Part model, mm, in its own coordinate system. Round coordinates to 2 decimals unless told otherwise and drop trailing zeros. Order: outer loops, then holes, each group sorted by start corner. A loop starts at its lowest first (then second) coordinate and runs counter-clockwise, first axis right, second up. Notation, with made-up numbers: (-6.75, 0) - (42.25, 0) arc R11 cw to (42.25, 10) - close; hole circle Ø6 at (2, 62.5). An arc over 180 degrees is marked (long way). Return JSON: item names as keys, results as strings. Group by question number.
Item 1: Probe probe 1 along Y at (x, z) = (425.45, 0.5); probe 2 along Y at (x, z) = (361.95, 0.85); probe 3 along X at (y, z) = (-7, 1.15). List the from-to ranges inside material, lowest first.
Item 2: Saw through at D-D on x = 404. List the corners of the cut face in (y, z), and give its area (3 significant figures).
Item 3: Two-plate mould, pull along Y, no slides. Class faces 1 (the face through (364.155, -6.613, 0.783)), 2 (the face through (410, 13, 1.588)), 3 (the face through (450.57, -7.61, 0.78)): released by +Y, released by -Y, zero draft, split by the parting line, or undercut.
Item 4: Saw through at C-C on z = 1.2. List the corners of the cut face in (x, y), and give its area (3 significant figures).
Item 5: Saw through at B-B on y = 20.65. List the corners of the cut face in (x, z).
Item 6: Saw through at A-A on x = 425.45. List the corners of the cut face in (y, z), and give its area (3 significant figures).
Autodesk Inventor part; units mm, degrees
ref_plane "YZ Plane" through (0, 0, 0) normal (1, 0, 0) x (0, 1, 0)
ref_plane "XZ Plane" through (0, 0, 0) normal (0, 1, 0) x (-1, 0, 0)
ref_plane "XY Plane" through (0, 0, 0) normal (0, 0, 1) x (1, 0, 0)
sketch "Sketch1" plane through (0, 0, 0) normal (0, 0, 1) x (1, 0, 0)
  circle A0 centre (425.45, 20.65) radius 2.0828
  circle A1 centre (425.45, 20.65) radius 34.925 construction
  line L0 (425.45, 55.575) -> (298.45, 55.575) construction
  line L1 (323.85, 55.575) -> (323.85, 42.875) construction
  circle A2 centre (323.85, 12.649) radius 30.226 construction
  circle A3 centre (425.45, 20.65) radius 33.02 construction
  line L2 (406.9994, 48.5755) -> (348.6303, -5.5907)
  line L3 (420.1242, 27) -> (481.5758, 27)
  line L4 (442.214, -11.1) -> (383.027, -11.1)
  line L5 (450.1296, -1.1362) -> (416.5451, 47.5277)
  circle A4 centre (425.45, 20.65) radius 7.9375 construction
  arc A5 (416.5451, 47.5277) -> (406.9994, 48.5755) centre (411.3189, 43.9209) ccw
  line L6 (444.9034, -11.093) -> (350.7901, -11.093)
  line L7 (457.0011, -11.093) -> (551.1145, -11.093) construction
  arc A6 (444.9034, -11.093) -> (450.1296, -1.1362) centre (444.9034, -4.743) ccw
  arc A7 (348.6303, -5.5907) -> (350.7901, -11.093) centre (350.7901, -7.918) ccw
  circle A8 centre (387.35, -5.9184) radius 2.3114
  circle A9 centre (361.95, -5.9184) radius 2.3114
  circle A10 centre (438.15, -5.9184) radius 2.3114
  circle A11 centre (425.45, -5.9184) radius 2.3368
  point P0 (0, 0)
  point P1 (342.7011, -11.093)
  dimension "d0" = 69.85
  dimension "d1" = 127
  dimension "d2" = 12.7
  dimension "d3" = 60.452
  dimension "d4" = 30.226
  dimension "d5" = 101.6
  dimension "d6" = 66.04
  dimension "d9" = 15.875
  dimension "d10" = 6.35
  dimension "d11" = 180
  dimension "d12" = 114.3
  dimension "d13" = 6.35
  dimension "d14" = 3.175
  dimension "d15" = 5.1746
  dimension "d16" = 101.6
  dimension "d19" = 4.6736
  dimension "d20" = 12.7
extrude "Extrusion1" add sketch "Sketch1" along normal blind 1.5875 contours A5 L5 A6 L6 A7 L2 | A8 | A10 | A11
extrude "Extrusion2" cut sketch "Sketch1" along normal blind 1.5875 contours A11
properties part number "tangentsled"
Filled in:
{
 "1": {"probe 1": "y = -11.09 to -8.26, -3.58 to 18.57, 22.73 to 34.62", "probe 2": "y = -11.09 to -8.23, -3.61 to 6.77", "probe 3": "x = 347.75 to 359.91, 363.99 to 423.38, 427.52 to 450.84"},
 "2": {"outline": "(-11.09, 0) - (45.79, 0) - (45.79, 1.59) - (-11.09, 1.59) - close", "area": "90.3 mm^2"},
 "3": {"face 1": "undercut", "face 2": "zero draft", "face 3": "split by the parting line"},
 "4": {"outline": "(348.63, -5.59) arc R3.18 ccw to (350.79, -11.09) - (444.9, -11.09) arc R6.35 ccw to (450.13, -1.14) - (416.55, 47.53) arc R6.35 ccw to (407, 48.58) - close; hole circle Ø4.62 at (361.95, -5.92); hole circle Ø4.67 at (425.45, -5.92); hole circle Ø4.17 at (425.45, 20.65)", "area": "3,590 mm^2"},
 "5": {"outline": "(376.91, 0) - (423.37, 0) - (423.37, 1.59) - (376.91, 1.59) - close; (427.53, 0) - (435.09, 0) - (435.09, 1.59) - (427.53, 1.59) - close"},
 "6": {"outline": "(-11.09, 0) - (-8.26, 0) - (-8.26, 1.59) - (-11.09, 1.59) - close; (-3.58, 0) - (18.57, 0) - (18.57, 1.59) - (-3.58, 1.59) - close; (22.73, 0) - (34.62, 0) - (34.62, 1.59) - (22.73, 1.59) - close", "area": "58.5 mm^2"}
}
